Could you check a few things on this model? Use its own coordinates, in mm. Face numbers are marked on the shaded views. Coordinates: 2 decimals unless noted, no trailing zeros. Order: outer loops, then holes, each group sorted by start corner. A loop starts at its lowest first (then second) coordinate and runs counter-clockwise, first axis right, second up. Notation, with made-up numbers: (-2.75, -36.75) -> (14.25, -36.75) arc R21 cw to (14.25, -21.75) -> close; hole circle Ø8 at (-7, -34.5). An arc over 180 degrees is marked (long way). Return JSON: item names as keys, results as strings. Group by question number.
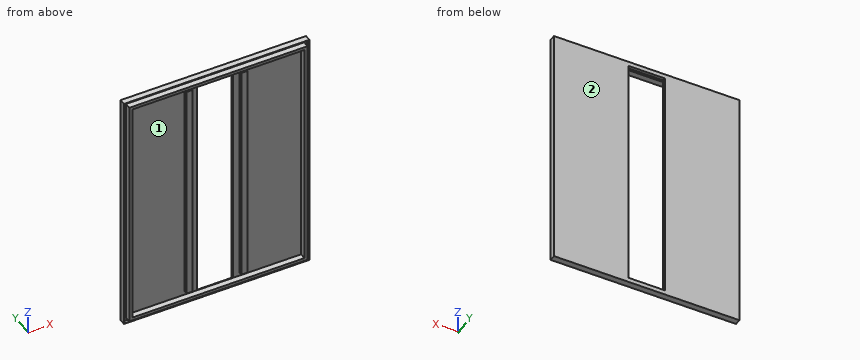
from build123d import *

# Parameters (mm, degrees)
SKETCH1_W           = 152.5
SKETCH1_H           = 202.5
BOSS_EXTRUDE1_DEPTH = 5
SKETCH3_W           = 151.5
SKETCH3_H           = 201.5
CUT_EXTRUDE1_DEPTH  = 2.5
SKETCH5_W           = 146.5
SKETCH5_H           = 196.5
SKETCH5_W_2         = 141.5
SKETCH5_H_2         = 191.5
BOSS_EXTRUDE3_DEPTH = 5
SKETCH6_W           = 30
SKETCH6_H           = 195
CUT_EXTRUDE4_DEPTH  = 2.5
SKETCH7_W           = 5
SKETCH7_H           = 185.5
BOSS_EXTRUDE5_DEPTH = 3


with BuildPart() as part:
    # Sketch1 → Boss-Extrude1 (new body)
    with BuildSketch(Plane(origin=(0, 0, 0), x_dir=(1, 0, 0), z_dir=(0, 1, 0))):
        Rectangle(SKETCH1_W, SKETCH1_H)
    extrude(amount=-BOSS_EXTRUDE1_DEPTH)

    # Sketch3 → Cut-Extrude1 (cut)
    with BuildSketch(Plane.XZ.offset(5)):
        Rectangle(SKETCH3_W, SKETCH3_H)
    extrude(amount=-CUT_EXTRUDE1_DEPTH, mode=Mode.SUBTRACT)

    # Sketch5 → Boss-Extrude3 (add)
    with BuildSketch(Plane.XZ.offset(2.5)):
        Rectangle(SKETCH5_W, SKETCH5_H)
        Rectangle(SKETCH5_W_2, SKETCH5_H_2, mode=Mode.SUBTRACT)
    extrude(amount=BOSS_EXTRUDE3_DEPTH)

    # Sketch6 → Cut-Extrude4 (cut)
    with BuildSketch(Plane(origin=(0, 0, 0), x_dir=(1, 0, 0), z_dir=(0, 1, 0))):
        Rectangle(SKETCH6_W, SKETCH6_H)
    extrude(amount=-CUT_EXTRUDE4_DEPTH, mode=Mode.SUBTRACT)

    # Sketch7 → Boss-Extrude5 (add)
    with BuildSketch(Plane.XZ.offset(2.5)):
        with Locations((-22.5, 0)):
            Rectangle(SKETCH7_W, SKETCH7_H)
        with Locations((22.5, 0)):
            Rectangle(SKETCH7_W, SKETCH7_H)
    extrude(amount=BOSS_EXTRUDE5_DEPTH)


solid = part.part
Q1. I want a section at C-C on z = -19. Please give me the cut outline in (x, y).
Q2. I need wall thicknesses on line 1 along Z through (x, y) = (-62, -3.5); line 2 along X through (y, z) = (-3.75, -40.5); line 3 along Z through (x, y) = (-23.5, -4.75). Which ranges of each line are inside material? Lowest first, please. Write a range as from..to.
Q3. We'd pull the mould along Z, two halves only. Please class the marked faces 1 and 2: pulls with the +Z half, pulls with the -Z half, needs draft (parallel to the pull), parting line crosses it, or undercut.
Q4. I'm going to push flat-ended pins straight in: pin 1 Ø5 at (x, z) = (-20.5, -24) entering from -Y; pin 2 Ø1.5 at (x, y) = (-32.5, -6.5) entering from +Z; pin 3 Ø0.5 at (x, z) = (-3.5, -96.5) entering from +Y. Where does each tip first touch, or does it pass through?
Q5. I want a section at D-D on x = -36. Please give me the cut outline in (y, z).
Q6. I want a section at B-B on y = -1.25. Please give me the cut outline in (x, z), and give its area (3 significant figures).
Q7. I want a section at A-A on x = -1. Please give me the cut outline in (y, z).
Response values:
{
 "1": {"outline": "(-76.25, -5) -> (-75.75, -5) -> (-75.75, -2.5) -> (-73.25, -2.5) -> (-73.25, -7.5) -> (-70.75, -7.5) -> (-70.75, -2.5) -> (-25, -2.5) -> (-25, -5.5) -> (-20, -5.5) -> (-20, -2.5) -> (-15, -2.5) -> (-15, 0) -> (-76.25, 0) -> close; (15, -2.5) -> (20, -2.5) -> (20, -5.5) -> (25, -5.5) -> (25, -2.5) -> (70.75, -2.5) -> (70.75, -7.5) -> (73.25, -7.5) -> (73.25, -2.5) -> (75.75, -2.5) -> (75.75, -5) -> (76.25, -5) -> (76.25, 0) -> (15, 0) -> close"},
 "2": {"line 1": "z = -101.25..-100.75, -98.25..-95.75, 95.75..98.25, 100.75..101.25", "line 2": "x = -76.25..-75.75, -73.25..-70.75, -25..-20, 20..25, 70.75..73.25, 75.75..76.25", "line 3": "z = -101.25..-100.75, -98.25..-95.75, -92.75..92.75, 95.75..98.25, 100.75..101.25"},
 "3": {"face 1": "undercut", "face 2": "needs draft"},
 "4": {"pin 1": "stops at y = -5.5", "pin 2": "stops at z = 98.25", "pin 3": "stops at y = -2.5"},
 "5": {"outline": "(-7.5, -98.25) -> (-2.5, -98.25) -> (-2.5, -100.75) -> (-5, -100.75) -> (-5, -101.25) -> (0, -101.25) -> (0, 101.25) -> (-5, 101.25) -> (-5, 100.75) -> (-2.5, 100.75) -> (-2.5, 98.25) -> (-7.5, 98.25) -> (-7.5, 95.75) -> (-2.5, 95.75) -> (-2.5, -95.75) -> (-7.5, -95.75) -> close"},
 "6": {"outline": "(-76.25, -101.25) -> (76.25, -101.25) -> (76.25, 101.25) -> (-76.25, 101.25) -> close; hole (-15, -97.5) -> (15, -97.5) -> (15, 97.5) -> (-15, 97.5) -> close", "area": "25,000 mm²"},
 "7": {"outline": "(-7.5, -98.25) -> (-2.5, -98.25) -> (-2.5, -100.75) -> (-5, -100.75) -> (-5, -101.25) -> (0, -101.25) -> (0, -97.5) -> (-2.5, -97.5) -> (-2.5, -95.75) -> (-7.5, -95.75) -> close; (-7.5, 95.75) -> (-2.5, 95.75) -> (-2.5, 97.5) -> (0, 97.5) -> (0, 101.25) -> (-5, 101.25) -> (-5, 100.75) -> (-2.5, 100.75) -> (-2.5, 98.25) -> (-7.5, 98.25) -> close"}
}
